Source: CAD feature listing. Evaluate the final solid. Frame: model axes, mm. Face numbers are marked on the shaded views. Give positions to 0.01 mm unless a question says otherwise; leave off trailing zeros. Loops run counter-clockwise (first coordinate to the right, second up) from the corner with the lowest first, then second, coordinate; pieces in that order, holes last. Notation, with made-up numbers: (-32.5, -32.5) -> (25.5, -32.5) arc R23 cw to (25.5, -7.5) -> close; hole circle Ø4 at (82.5, 22). An arc over 180 degrees is marked (long way). Return JSON: item names as keys, results as strings. Group by question number.
(1) Cut plane A-A on x = 0. Return loops of the section in (y, z).
(2) Cut plane B-B on z = 0. Return loops of the section in (x, y).
(3) Pin query (flat end, axial travel): pin 1 (2.5 mm diameter, centred on x = 0, z = 0, fed in from +Y); pin 2 (3 mm diameter, centred on x = 2, y = -3.5, fed in from -Z); pin 3 (3 mm diameter, centred on x = 2.5, y = -7, fed in from +Z); pin 4 (3 mm diameter, centred on y = -3, z = -0.5, fed in from -X). Return the tip coordinate at first contact, or that it passes through.
(4) Draft query along X for the marked faces 1, 2 and 3. Return one class per face: released by +X, released by -X, zero draft, split by the parting line, or undercut.
(5) Cut plane C-C on y = -1.5. Return loops of the section in (x, z).
(6) Ray query, line 1 (Z direction, x = 0, y = -4); line 2 (X direction, y = -7.25, z = -1); line 3 (Y direction, x = 0.5, z = -1.75). Return the intervals inside material, ascending. Write a range as from..to.
(7) Cut plane D-D on y = -7.75. Return loops of the section in (x, z).
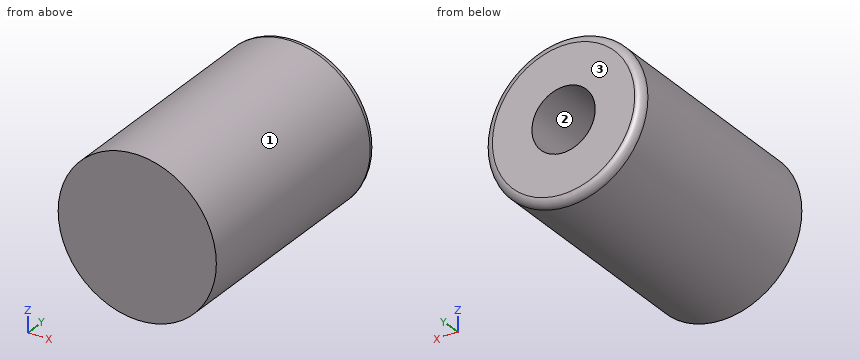
```python
from build123d import *

# Parameters (mm, degrees)
F0_R     = 5
F1_DEPTH = 15
F2_R     = 0.5
F3_R     = 2
F4_DEPTH = 7.5


with BuildPart() as f1:
    # F0 (on Front) → F1 (new body)
    with BuildSketch(Plane.XZ):
        Circle(F0_R)
    extrude(amount=F1_DEPTH)

    # F2
    f2_edges = [f1.edges().sort_by_distance(p)[0] for p in [
        (-5, 0, 0),
    ]]
    fillet(f2_edges, radius=F2_R)

    # F3 (on face) → F4 (cut)
    with BuildSketch(Plane(origin=(0, 0, 0), x_dir=(-1, 0, 0), z_dir=(0, 1, 0))):
        Circle(F3_R)
    extrude(amount=-F4_DEPTH, mode=Mode.SUBTRACT)


solid = f1.part
```
Answers:
{
 "1": {"outline": "(-15, -5) -> (-0.5, -5) arc R0.5 ccw to (0, -4.5) -> (0, -2) -> (-7.5, -2) -> (-7.5, 2) -> (0, 2) -> (0, 4.5) arc R0.5 ccw to (-0.5, 5) -> (-15, 5) -> close"},
 "2": {"outline": "(-5, -15) -> (5, -15) -> (5, -0.5) arc R0.5 ccw to (4.5, 0) -> (2, 0) -> (2, -7.5) -> (-2, -7.5) -> (-2, 0) -> (-4.5, 0) arc R0.5 ccw to (-5, -0.5) -> close"},
 "3": {"pin 1": "y = -7.5", "pin 2": "z = -4.97", "pin 3": "z = 4.9", "pin 4": "x = -5"},
 "4": {"face 1": "split by the parting line", "face 2": "undercut", "face 3": "zero draft"},
 "5": {"outline": "circle Ø10 at (0, 0); hole circle Ø4 at (0, 0)"},
 "6": {"line 1": "-5..-2, 2..5", "line 2": "-4.9..-1.73, 1.73..4.9", "line 3": "-15..-7.5"},
 "7": {"outline": "circle Ø10 at (0, 0)"}
}
